Geometry check sheet. Reference: the model listing, model coordinates, mm. A direction names the side the tool comes from. Round coordinates to 2 decimals unless told otherwise and drop trailing zeros. Loops run counter-clockwise (first coordinate to the right, second up) from the corner with the lowest first, then second, coordinate; pieces in that order, holes last. Notation, with made-up numbers: (67.5, 24.5) -> (108.5, 24.5) arc R26 ccw to (108.5, 52.5) -> close; hole circle Ø11 at (17, 47). An arc over 180 degrees is marked (long way). Use a Markdown table: item, result. Add a question column.
Q1. Material ranges on L1, parallel to Z at x = 7.5, y = 34.5; L2, parallel to Z at x = 7, y = 34; L3, parallel to Y at x = -1.5, z = 12, recorded low to high.
Q2. Release check for a two-part mould opening along X. For faces 1 (the face through (0, 9, 23.555)), 2 (the face through (-16.5, 35.55, -0.07)), 3 (the face through (5.344, 41.465, 8.381)), 4 (the face through (7, 32, -13)) record: released by +X, released by -X, zero draft, split by the parting line, or undercut.
Q3. Sectioned sample at B-B, the plane x = 0. Enter the section's corners in (y, z) (3 decimals).
Q4. Sectioned sample at D-D, the plane z = -6. Enter the section's corners in (x, y), then the cut area to 3 significant figures.
Q5. Gauge pin test, flat ends, axial feed: P1, Ø1, axis at x = -11.5, z = -4, coming from the +Y side; P2, Ø2, axis at y = 23, z = 5.5, coming from the -X side; P3, Ø3, axis at x = -5.5, y = 51.5, coming from the +Z side; P4, Ø2.5, axis at x = -15, z = 0, coming from the +Y side. Record the tip position at first contact, or that the pin passes through.
Q6. Sectioned sample at C-C, the plane y = 8.45. Enter the section's corners in (x, z) (3 decimals), then the cut area to 3 significant figures.
Q7. Set-up check for faces 5 (the face through (9.2, 39, -4.2)), 6 (the face through (0, 0, 0)), 7 (the face through (2, 54, 0)), 8 (the face through (-1, 59, 0)), 9 (the face through (-4.146, 8.632, 21.615)): record each of +Z, -Z, +X, -X, +Y, -Y from which the full face is reachable in a straight line by a thin tool's end or side.
Q8. Sectioned sample at A-A, the plane z = 0. Enter the section's corners in (x, y) (3 decimals), then the cut area to 3 significant figures.
Autodesk Inventor part; units mm, degrees
ref_plane "工作平面2" through (0, 0, 20) normal (0, 0, 1) x (1, 0, 0)
ref_plane "YZ Plane" through (0, 0, 0) normal (1, 0, 0) x (0, 1, 0)
ref_plane "XZ Plane" through (0, 0, 0) normal (0, 1, 0) x (-1, 0, 0)
sketch "草圖1" plane through (0, 0, 0) normal (0, 1, 0) x (-1, 0, 0)
  circle A0 centre (0, 0) radius 20.055
  dimension "d0" = 40.11
extrude "擠出1" add sketch "草圖1" along normal blind 39
sketch "草圖2" plane through (0, 39, 0) normal (0, 1, 0) x (1, 0, 0)
  circle A0 centre (0, 0) radius 9.94
  dimension "d3" = 19.88
extrude "擠出2" add sketch "草圖2" along normal blind 5
sketch "草圖3" plane through (0, 44, 0) normal (0, 1, 0) x (1, 0, 0)
  circle A0 centre (0, 0) radius 3
  dimension "d6" = 6
extrude "擠出3" add sketch "草圖3" along normal blind 15
sketch "草圖4" plane through (0, 59, 0) normal (0, 1, 0) x (1, 0, 0)
  circle A0 centre (0, 0) radius 3
  line L0 (-16.4783, -20) -> (15.8218, -20) construction
  line L1 (2, 2.2361) -> (2, -2.2361)
  arc A1 (2, -2.2361) -> (2, 2.2361) centre (0, 0) ccw
  point P0 (-3, 0)
  dimension "d9" = 20
  dimension "d10" = 20
  dimension "d11" = 5
extrude "擠出4" cut sketch "草圖4" against normal blind 10 contours A0 L1 picked at (2.1409, -0.5898)
ref_plane "工作平面2" through (0, 0, 20) normal (0, 0, 1) x (1, 0, 0)
sketch "草圖5" plane through (0, 0, 20) normal (0, 0, 1) x (1, 0, 0)
  circle A0 centre (0, 8.45) radius 4.15
  point P0 (0, 0)
  dimension "d16" = 8.3
  dimension "d17" = 8.45
extrude "擠出5" add sketch "草圖5" along normal mid plane 7.11
sketch "草圖6" plane through (0, 39, 0) normal (0, 1, 0) x (1, 0, 0)
  circle A0 centre (-15, 0) radius 1.5
  circle A1 centre (7.5, -12.9904) radius 1.5
  circle A2 centre (7.5, 12.9904) radius 1.5
  line L0 (0, 0) -> (7.5, -12.9904) construction
  arc A3 (2, 2.2361) -> (2, -2.2361) centre (0, 0) ccw
  line L1 (0, 0) -> (7.5, 12.9904) construction
  line L2 (0, 0) -> (-20.055, 0) construction
  circle A4 centre (0, 0) radius 20.055
  dimension "d20" = 120
  dimension "d21" = 120
  dimension "d22" = 3
  dimension "d23" = 15
  dimension "d24" = 15
  dimension "d25" = 15
extrude "擠出6" cut sketch "草圖6" against normal blind 7 contours A0 | A1 | A2
properties part number "E6B2-CWZ6C"
Values:
| question | item | result |
|---|---|---|
| 1 | L1 | -18.6 to -14.49, -11.49 to 11.49, 14.49 to 18.6 |
| 1 | L2 | -18.79 to -14.4, -11.58 to 11.58, 14.4 to 18.79 |
| 1 | L3 | 0 to 39 |
| 2 | face 1 | zero draft |
| 2 | face 2 | undercut |
| 2 | face 3 | split by the parting line |
| 2 | face 4 | undercut |
| 3 | outline | (0, -20.055) -> (39, -20.055) -> (39, -9.94) -> (44, -9.94) -> (44, -3) -> (59, -3) -> (59, 3) -> (44, 3) -> (44, 9.94) -> (39, 9.94) -> (39, 20.055) -> (12.6, 20.055) -> (12.6, 23.555) -> (4.3, 23.555) -> (4.3, 20.055) -> (0, 20.055) -> close |
| 4 | outline | (-19.14, 0) -> (19.14, 0) -> (19.14, 39) -> (7.92, 39) -> (7.92, 44) -> (-7.92, 44) -> (-7.92, 39) -> (-19.14, 39) -> close |
| 4 | area | 1,570 mm^2 |
| 5 | P1 | y = 39 |
| 5 | P2 | x = -19.54 |
| 5 | P3 | through |
| 5 | P4 | y = 32 |
| 6 | outline | (-4.15, 19.621) arc R20.055 ccw (long way) to (4.15, 19.621) -> (4.15, 23.555) -> (-4.15, 23.555) -> close |
| 6 | area | 1,290 mm^2 |
| 7 | face 5 | +Y |
| 7 | face 6 | +Z, -Z, +X, -X, -Y |
| 7 | face 7 | +Z, -Z, +X, +Y |
| 7 | face 8 | +Z, -Z, +X, -X, +Y |
| 7 | face 9 | +Z |
| 8 | outline | (-20.055, 0) -> (20.055, 0) -> (20.055, 39) -> (9.94, 39) -> (9.94, 44) -> (3, 44) -> (3, 49) -> (2, 49) -> (2, 59) -> (-3, 59) -> (-3, 44) -> (-9.94, 44) -> (-9.94, 39) -> (-13.5, 39) -> (-13.5, 32) -> (-16.5, 32) -> (-16.5, 39) -> (-20.055, 39) -> close |
| 8 | area | 1,720 mm^2 |
